Check sheet for the drawn part. Datum: minimum x, y, z corner. Units: mm. Give positions to 0.01 mm unless a question says otherwise; leave off trailing zeros. Write each loop counter-clockwise with the first axis right and the second up, starting at its lowest first coordinate (ties: lowest second). Pieces come first, ordered by that corner, then holes. Notation, with made-up numbers: M 38,-8.5 L 60,-8.5 A20 cw 60,11.5 Z; hole C 1,-11 d8. An arc over 180 degrees is marked long. Write item = value, one per line. Start each with the question number.
1) Sectioned sample at C-C, the plane x = 4. Record the cut outline in (y, z).
2) Sectioned sample at B-B, the plane z = 5. Record the cut outline in (x, y) (1 decimal).
3) Sectioned sample at A-A, the plane x = 19.5. Count the separate pieces of the cut face and the enclosed holes in it, then the cut area to 3 significant figures.
4) Gauge pin test, flat end, axial feed: pin 1 (3 mm diameter, centred on x = 3.58, y = 4.6, fed in from -Z). Record the tip position at first contact, or that the pin passes through.
5) Draft check along X on the marked faces 1, 2 and 3. Enter one of: pulls with the +X half, pulls with the -X half, needs draft (parallel to the pull), parting line crosses it, or undercut.
6) Scan lines: L1, parallel to X at y = 28, z = 9.5 (1 decimal); L2, parallel to Y at x = 16.75, z = 1 (1 decimal); L3, parallel to Y at x = 3, z = 2.5 (1 decimal). Record each from-to range of solid material in increasing order.
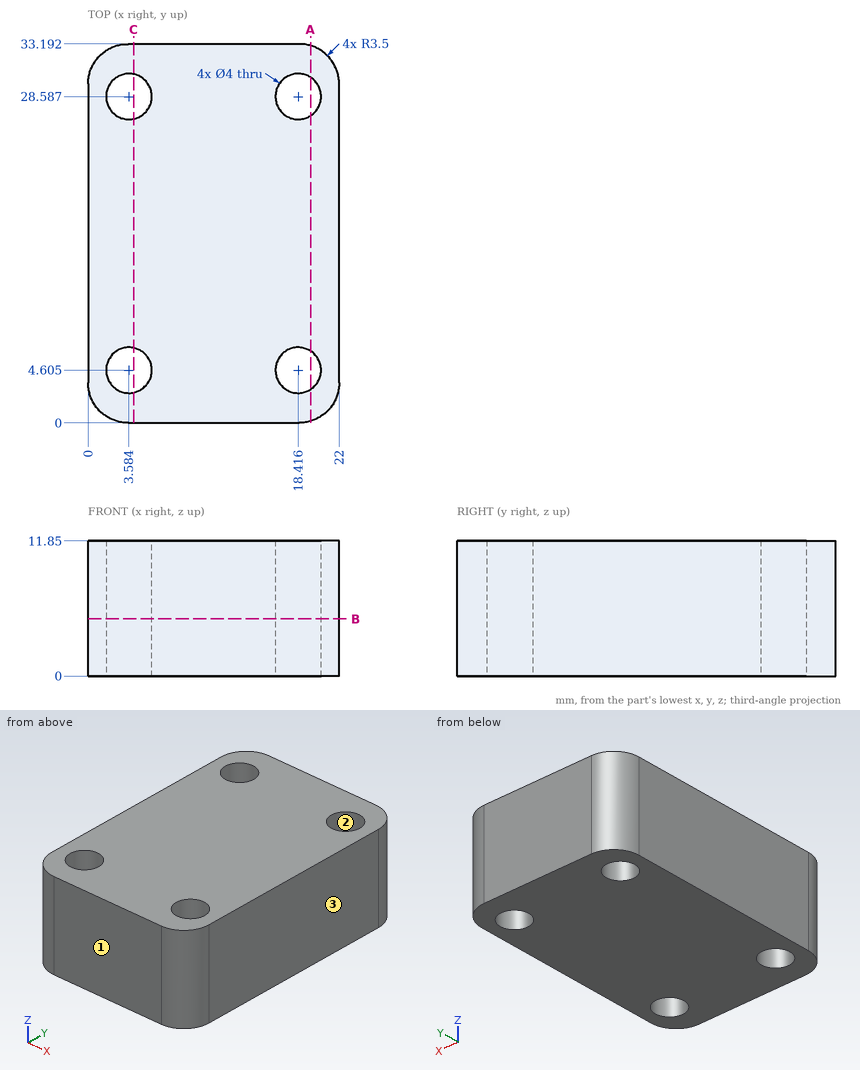
Data:
q1.outline = M 0,0 L 2.65,0 L 2.65,11.85 L 0,11.85 Z; M 6.56,0 L 26.63,0 L 26.63,11.85 L 6.56,11.85 Z; M 30.54,0 L 33.19,0 L 33.19,11.85 L 30.54,11.85 Z
q2.outline = M 0,3.5 A3.5 ccw 3.5,0 L 18.5,0 A3.5 ccw 22,3.5 L 22,29.7 A3.5 ccw 18.5,33.2 L 3.5,33.2 A3.5 ccw 0,29.7 Z; hole C 3.6,4.6 d4; hole C 3.6,28.6 d4; hole C 18.4,4.6 d4; hole C 18.4,28.6 d4
q3.separate_pieces = 3
q3.enclosed_holes = 0
q3.area = 310 mm2
q4.pin_1 = through
q5.face_1 = needs draft
q5.face_2 = undercut
q5.face_3 = pulls with the +X half
q6.L1 = 0 to 1.7, 5.5 to 16.5, 20.3 to 22
q6.L2 = 0 to 3.5, 5.7 to 27.5, 29.7 to 33.2
q6.L3 = 0 to 2.7, 6.5 to 26.7, 30.5 to 33.2
